Can you work these out from the model? Positions are in its coordinate system, mm. Give positions to 0.01 mm unless a question says otherwise; leave off trailing zeros. Write each loop counter-clockwise with the first axis right and the second up, starting at its lowest first coordinate (ties: lowest second). Pieces come first, ordered by that corner, then holes.
Autodesk Inventor part; units mm, degrees
ref_plane "YZ Plane" through (0, 0, 0) normal (1, 0, 0) x (0, 1, 0)
ref_plane "XZ Plane" through (0, 0, 0) normal (0, 1, 0) x (-1, 0, 0)
ref_plane "XY Plane" through (0, 0, 0) normal (0, 0, 1) x (1, 0, 0)
sketch "Sketch1" plane through (0, 0, 0) normal (0, 0, 1) x (1, 0, 0)
  line L0 (0, 0) -> (160, 0)
  line L1 (160, 0) -> (160, 50)
  line L2 (160, 50) -> (0, 50)
  line L3 (0, 50) -> (0, 0)
  line L4 (0, 0) -> (21, 0)
  circle A0 centre (21, 35) radius 3.25
  circle A1 centre (21, 15) radius 3.25
  circle A2 centre (139, 15) radius 3.25
  circle A3 centre (139, 35) radius 3.25
  circle A4 centre (80, 15) radius 6.35
  point P0 (80, 25)
  point P1 (80, 25)
  point P2 (80, 50)
  dimension "d0" = 160
  dimension "d1" = 50
  dimension "d2" = 21
  dimension "d5" = 6.5
  dimension "d6" = 6.5
  dimension "d13" = 20
  dimension "d14" = 15
  dimension "d15" = 21
  dimension "d19" = 360
  dimension "d23" = 80
  dimension "d24" = 12.7
  dimension "d25" = 35
extrude "Extrusion1" add sketch "Sketch1" along normal blind 6 contours L3 L2 L1 L0 | A0 | A2 | A3 | A4
extrude "Extrusion3" cut sketch "Sketch1" along normal blind 10 contours A0 | A2 | A3 | A4
sketch "Sketch4" plane through (0, 50, 0) normal (0, 1, 0) x (1, 0, 0)
  point P0 (0, 0)
properties part number "support plate 2"
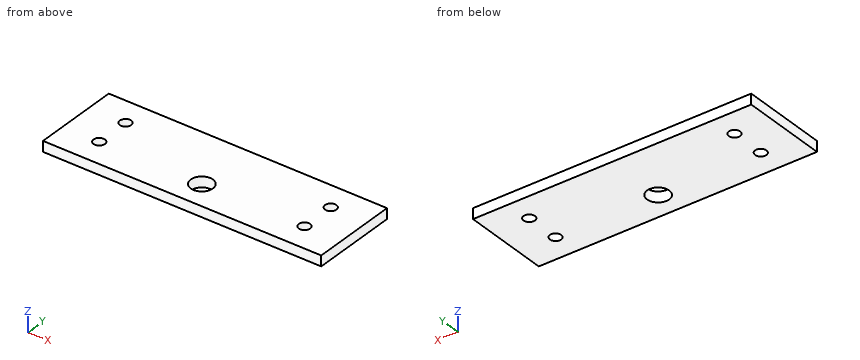
(1) Will these pins go through, and if not, where does the flat tip stop? P1, Ø1, axis at y = 38.5, z = 5, coming from the -X side; P2, Ø6, axis at x = 21, y = 35, coming from the +Z side.
Returned:
P1: stops at x = 0
P2: passes through
(2) Imagine slicing it at D-D, the plane x = 22.5. Write out the boundary of the cut face in (y, z).
Returned:
outline: (0, 0) - (12.12, 0) - (12.12, 6) - (0, 6) - close; (17.88, 0) - (32.12, 0) - (32.12, 6) - (17.88, 6) - close; (37.88, 0) - (50, 0) - (50, 6) - (37.88, 6) - close
(3) Imagine slicing it at B-B, the plane x = 80. Write out the boundary of the cut face in (y, z).
Returned:
outline: (0, 0) - (8.65, 0) - (8.65, 6) - (0, 6) - close; (21.35, 0) - (50, 0) - (50, 6) - (21.35, 6) - close
(4) Imagine slicing it at C-C, the plane z = 2.85. Write out the boundary of the cut face in (x, y), plus the area to 3 significant figures.
Returned:
outline: (0, 0) - (160, 0) - (160, 50) - (0, 50) - close; hole circle Ø6.5 at (21, 15); hole circle Ø6.5 at (21, 35); hole circle Ø12.7 at (80, 15); hole circle Ø6.5 at (139, 15); hole circle Ø6.5 at (139, 35)
area: 7,740 mm2
(5) Imagine slicing it at A-A, the plane x = 139. Write out the boundary of the cut face in (y, z).
Returned:
outline: (0, 0) - (11.75, 0) - (11.75, 6) - (0, 6) - close; (18.25, 0) - (31.75, 0) - (31.75, 6) - (18.25, 6) - close; (38.25, 0) - (50, 0) - (50, 6) - (38.25, 6) - close
(6) If I drill on L1, parallel to Y at x = 21, z = 2.2; L2, parallel to X at y = 35, z = 2.2; L3, parallel to Y at x = 80, z = 4.3, over which ranges is the centre line in solid material (lowest first)?
Returned:
L1: y = 0 to 11.75, 18.25 to 31.75, 38.25 to 50
L2: x = 0 to 17.75, 24.25 to 135.75, 142.25 to 160
L3: y = 0 to 8.65, 21.35 to 50
